CAD build for the part. Positions are in the model's coordinates, mm. Face numbers are marked on the shaded views. A direction names the side the tool comes from. Give positions to 0.01 mm unless a question says otherwise; leave off trailing zeros. Order: outer loops, then holes, each group sorted by start corner. A loop starts at its lowest first (then second) coordinate and runs counter-clockwise, first axis right, second up.
from build123d import *

# Parameters (mm, degrees)
SKETCH1_R                                        = 5
BOSS_EXTRUDE1_DEPTH                              = 30
SKETCH2_W                                        = 160
SKETCH2_H                                        = 30
BOSS_EXTRUDE2_DEPTH                              = 10
RIB1_REACH                                       = 529.146
SKETCH5_WALL_W                                   = 1084.577110596
SKETCH5_WALL_H                                   = 10
RIB17_REACH                                      = 529.146
SKETCH7_WALL_W                                   = 1084.577110596
SKETCH7_WALL_H                                   = 10
CBORE_FOR_M4_HEX_HEAD_MACHINE_SCREW2_D           = 4.5
CBORE_FOR_M4_HEX_HEAD_MACHINE_SCREW2_CBORE_D     = 10.59
CBORE_FOR_M4_HEX_HEAD_MACHINE_SCREW2_CBORE_DEPTH = 3
MIRROR2_COPY_1_D                                 = 4.5
MIRROR2_COPY_1_CBORE_D                           = 10.59
MIRROR2_COPY_1_CBORE_DEPTH                       = 3
BOSS_EXTRUDE5_DEPTH                              = 90
CUT_EXTRUDE4_DEPTH                               = 100
CUT_EXTRUDE4_DEPTH_BACK                          = 100


with BuildPart() as part:
    # Sketch1 → Boss-Extrude1 (new body)
    with BuildSketch(Plane.XY):
        with BuildLine():
            Line((-7.071067812, 7.071067812), (75.857864376, 90))
            Line((75.857864376, 90), (375.857864376, 90))
            ThreePointArc((375.857864376, 90), (411.213203436, 75.355339059), (425.857864376, 40))
            Line((425.857864376, 40), (425.857864376, -260))
            Line((425.857864376, -260), (325.857864376, -360))
            Line((325.857864376, -360), (325.857864376, -410))
            Line((325.857864376, -410), (205.857864376, -400))
            Line((205.857864376, -400), (205.857864376, -380))
            Line((205.857864376, -380), (295.857864376, -380))
            Line((295.857864376, -380), (295.857864376, -300))
            Line((295.857864376, -300), (335.857864376, -260))
            Line((335.857864376, -260), (335.857864376, -60))
            ThreePointArc((335.857864376, -60), (321.213203436, -24.644660941), (285.857864376, -10))
            Line((285.857864376, -10), (0, -10))
            ThreePointArc((0, -10), (-9.238795325, -3.826834324), (-7.071067812, 7.071067812))
        make_face()
        Circle(SKETCH1_R, mode=Mode.SUBTRACT)
    extrude(amount=BOSS_EXTRUDE1_DEPTH)

    # Sketch2 → Boss-Extrude2 (add)
    with BuildSketch(Plane.XZ.offset(10)):
        with Locations((100, 45)):
            Rectangle(SKETCH2_W, SKETCH2_H)
        with Locations((100, 15)):
            Rectangle(SKETCH2_W, SKETCH2_H)
        with Locations((100, -15)):
            Rectangle(SKETCH2_W, SKETCH2_H)
    extrude(amount=BOSS_EXTRUDE2_DEPTH)

    # Sketch5 wall → Rib1 (add, up to next)
    with BuildSketch(Plane(origin=(100, 0, 40), x_dir=(0, -0.707106781187, 0.707106781187), z_dir=(0, 0.707106781187, 0.707106781187)), mode=Mode.PRIVATE) as rib1_sk1:
        Rectangle(SKETCH5_WALL_W, SKETCH5_WALL_H)
    rib1_tool1 = extrude(rib1_sk1.sketch, amount=-RIB1_REACH, mode=Mode.PRIVATE) - part.part
    add(rib1_tool1.solids().sort_by_distance((100, 0, 40))[0])

    # Sketch7 wall → Rib17 (add, up to next)
    with BuildSketch(Plane(origin=(100, 0, -10), x_dir=(0, -0.707106781187, -0.707106781187), z_dir=(0, -0.707106781187, 0.707106781187)), mode=Mode.PRIVATE) as rib17_sk1:
        Rectangle(SKETCH7_WALL_W, SKETCH7_WALL_H)
    rib17_tool1 = extrude(rib17_sk1.sketch, amount=RIB17_REACH, mode=Mode.PRIVATE) - part.part
    add(rib17_tool1.solids().sort_by_distance((100, 0, -10))[0])

    # CBORE for M4 Hex Head Machine Screw2 (through all)
    with Locations(Plane(origin=(0, -10, 0), x_dir=(1, 0, 0), z_dir=(0, 1, 0))):
        with Locations((130, -48.5), (150, -48.5), (170, -48.5)):
            cbore_for_m4_hex_head_machine_screw2 = CounterBoreHole(CBORE_FOR_M4_HEX_HEAD_MACHINE_SCREW2_D / 2, CBORE_FOR_M4_HEX_HEAD_MACHINE_SCREW2_CBORE_D / 2, CBORE_FOR_M4_HEX_HEAD_MACHINE_SCREW2_CBORE_DEPTH)

    # Mirror1: CBORE for M4 Hex Head Machine Screw2 across plane
    add(cbore_for_m4_hex_head_machine_screw2.mirror(Plane(origin=(100, 0, 0), x_dir=(0, 0, 1), z_dir=(1, 0, 0))), mode=Mode.SUBTRACT)

    # Mirror2: CBORE for M4 Hex Head Machine Screw2 across plane
    add(cbore_for_m4_hex_head_machine_screw2.mirror(Plane.XY.offset(16)), mode=Mode.SUBTRACT)

    # Mirror2 copy 1 (through all)
    with Locations(Plane(origin=(200, -10, 32), x_dir=(-1, 0, 0), z_dir=(0, 1, 0))):
        with Locations((130, -48.5), (150, -48.5), (170, -48.5)):
            CounterBoreHole(MIRROR2_COPY_1_D / 2, MIRROR2_COPY_1_CBORE_D / 2, MIRROR2_COPY_1_CBORE_DEPTH)

    # Sketch19 → Boss-Extrude5 (add)
    with BuildSketch(Plane.ZY.offset(-295.857864376)):
        with BuildLine():
            Line((-23.890872965, -394.024153256), (-16.819805153, -401.095221068))
            ThreePointArc((-16.819805153, -401.095221068), (15, -387.915026221), (46.819805153, -401.095221068))
            Line((46.819805153, -401.095221068), (53.890872965, -394.024153256))
            ThreePointArc((53.890872965, -394.024153256), (15, -377.915026221), (-23.890872965, -394.024153256))
        make_face()
    extrude(amount=BOSS_EXTRUDE5_DEPTH)

    # Sketch20 → Cut-Extrude4 (cut, two sides: drawn at the far end of the back side and taken through both)
    with BuildSketch(Plane(origin=(-31.683738866, -380.204866396, 0), x_dir=(0.9965457582448797, -0.08304547985374006, 0), z_dir=(-0.08304547985374006, -0.9965457582448797, 0)).offset(-CUT_EXTRUDE4_DEPTH_BACK)):
        Polygon((228.178842993, -32.182148517), (344.185851358, -32.182148517), (238.364973487, 0), (228.178842993, 3.097796682), align=None)
        Polygon((238.364973487, 30), (346.499317462, 62.242718318), (228.178842993, 62.242718318), (228.178842993, 26.962773119), align=None)
    extrude(amount=CUT_EXTRUDE4_DEPTH + CUT_EXTRUDE4_DEPTH_BACK, mode=Mode.SUBTRACT)


solid = part.part
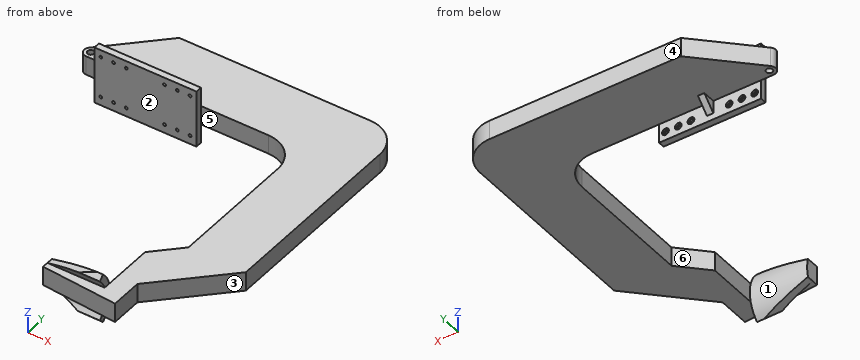
1. Saw through at C-C on y = -284. Give the cut face in (x, z), plus the area to 3 significant figures.
2. Saw through at A-A on z = 7.5. Give the cut face in (x, y).
3. Saw through at B-B on x = 215. Give the cut face in (y, z), plus the area to 3 significant figures.
4. Pin check, flat tips, straight feed: P1, Ø17, axis at x = 50, z = 48.5, coming from the -Y side; P2, Ø3, axis at y = -11.5, z = 45, coming from the -X side; P3, Ø15, axis at y = -374, z = 20, coming from the +X side; P4, Ø2.5, axis at x = 70, z = -16.5, coming from the -Y side. Stop position of each tip, or through.
5. Mould opens along X. For the marked faces 4, 5 and 6 say: released by +X, released by -X, zero draft, split by the parting line, or undercut.
6. Wall check: line 1 (Z direction, x = 50, y = -11.4) (3 decimals); line 2 (Z direction, x = 150, y = -16); line 3 (Y direction, x = 83, z = 19). Give the ranges that are in metal, low to high.
7. Saw through at D-D on x = 386.5. Give the cut face in (y, z), plus the area to 3 significant figures.
8. 3-axis set-ups, long thin cutter, end or side, ignore diameter. For the marked faces 1, 2 and 3: which of +Z, -Z, +X, -X, +Y, -Y reach the whole face in a straight line?
Reported:
1. outline: (311.86, 0) - (401.86, 0) - (401.86, 30) - (311.86, 30) - close
1. area: 2,700 mm2
2. outline: (-7.07, 7.07) arc R10 ccw to (0, -10) - (20, -10) - (20, -20) - (180, -20) - (180, -10) - (285.86, -10) arc R50 cw to (335.86, -60) - (335.86, -260) - (295.86, -300) - (295.86, -378.43) - (205.86, -378.43) - (205.86, -400) - (325.86, -410) - (325.86, -360) - (425.86, -260) - (425.86, 40) arc R50 ccw to (375.86, 90) - (75.86, 90) - close; hole circle Ø10 at (0, 0)
3. outline: (-400.76, 0) - (-390.49, 0) arc R45 cw to (-391.48, -2.56) - (-380.7, -2.28) arc R55 ccw to (-380.69, 32.24) - (-391.46, 32.51) arc R45 cw to (-390.49, 30) - (-400.76, 30) - close; (-10, 0) - (90, 0) - (90, 30) - (-10, 30) - close
3. area: 3,720 mm2
4. P1: stops at y = -20
4. P2: stops at x = 20
4. P3: stops at x = 325.86
4. P4: passes through
5. face 4: zero draft
5. face 5: undercut
5. face 6: released by -X
6. line 1: z = -30 to -21.795, -11.205 to 43.205, 53.795 to 60
6. line 2: z = -30 to -18.75, -14.25 to 46.25, 50.75 to 60
6. line 3: y = -20 to 90
7. outline: (-299.36, 0) - (88.85, 0) - (88.85, 30) - (-299.36, 30) - close
7. area: 11,600 mm2
8. face 1: -X
8. face 2: +Z, -Z, -X, -Y
8. face 3: +Z, -Z, +X, -Y
